from build123d import *

# Parameters (mm, degrees)
SKETCH_1_R      = 65
SKETCH_1_R_2    = 54
EXTRUDE_1_DEPTH = 50
FILLET_1_R      = 8
SHELL_1_T       = -4


with BuildPart() as part:
    # Эскиз1 → Вытянуть-Тонкостенный1 (new body)
    with BuildSketch(Plane.XY):
        Circle(SKETCH_1_R)
        Circle(SKETCH_1_R_2, mode=Mode.SUBTRACT)
    extrude(amount=EXTRUDE_1_DEPTH)

    # Скругление1
    fillet_1_edges = [part.edges().sort_by_distance(p)[0] for p in [
        (-65, 0, 0),
        (-65, 0, 50),
    ]]
    fillet(fillet_1_edges, radius=FILLET_1_R)

    # Оболочка1
    shell_1_openings = [part.faces().sort_by_distance(p)[0] for p in [
        (-54, 0, 25),
    ]]
    offset(amount=SHELL_1_T, openings=shell_1_openings, kind=Kind.INTERSECTION)


solid = part.part
For this review, take the finished solid that the model builds, in its own axes (mm). A direction names the side the tool comes from. Coordinates: 2 decimals unless noted, no trailing zeros. Write each loop counter-clockwise with the first axis right and the second up, starting at its lowest first coordinate (ties: lowest second). Pieces come first, ordered by that corner, then holes. Notation, with made-up numbers: (69.25, -25.75) -> (128.25, -25.75) arc R8 cw to (128.25, -15.75) -> close; hole circle Ø6 at (26.5, 1.25). An arc over 180 degrees is marked (long way). Write each question's results on one line, items separated by ' | '. Start each with the question number.
1) Consider section A-A (y = 0). Write out the cut boundary in (x, z), plus the area to 3 significant figures.
2) Wall thickness on L1, parallel to Y at x = 0, z = 34.5; L2, parallel to Z at x = -29.5, y = 47.5; L3, parallel to X at y = 50.5, z = 32.5: over which ranges is each line inside the solid? List them lowest first. Write a range as [from, to].
3) Consider section C-C (z = 37). Write out the cut boundary in (x, y).
4) The part is to be moulded in two halves that separate along Z. For faces 3 (the face through (50, -21, 50)), 4 (the face through (-48.408, -37.118, 24.762)), 5 (the face through (50, -21, 46)), 6 (the face through (-11.706, -52.716, 1.972)), say which applies: +Z half, -Z half, draft (parallel to the pull), parting line (faces both ways), or undercut.
5) For faces 1 (the face through (50, -21, 0)), 2 (the face through (50, -21, 4)), list the 3-axis set-ups (+Z, -Z, +X, -X, +Y, -Y) from which the entire face can be reached by the end or side of a thin tool; tool diameter is ignored.
6) Insertion check: pin 1 (10 mm diameter, centred on x = 2, z = 14.5, fed in from +Y); pin 2 (2 mm diameter, centred on y = -39, z = 35, fed in from -X); pin 3 (8 mm diameter, centred on y = 39, z = 34, fed in from +X). Each pin has a flat end and moves straight along its axis. Give the tip position at first contact, or say it passes through.
Geometry says:
1) outline: (-65, 8) arc R8 ccw to (-57, 0) -> (-54, 0) -> (-54, 4) -> (-57, 4) arc R4 cw to (-61, 8) -> (-61, 42) arc R4 cw to (-57, 46) -> (-54, 46) -> (-54, 50) -> (-57, 50) arc R8 ccw to (-65, 42) -> close; (54, 0) -> (57, 0) arc R8 ccw to (65, 8) -> (65, 42) arc R8 ccw to (57, 50) -> (54, 50) -> (54, 46) -> (57, 46) arc R4 cw to (61, 42) -> (61, 8) arc R4 cw to (57, 4) -> (54, 4) -> close | area: 471 mm^2
2) L1: [-65, -61], [61, 65] | L2: [0, 4], [46, 50] | L3: [-40.92, -34.22], [34.22, 40.92]
3) outline: circle Ø130 at (0, 0); hole circle Ø122 at (0, 0)
4) face 3: +Z half | face 4: undercut | face 5: undercut | face 6: draft
5) face 1: -Z, +X, -X, +Y, -Y | face 2: none
6) pin 1: y = 65 | pin 2: x = -52.74 | pin 3: x = 54.77
